Autodesk Inventor part; units mm, degrees
ref_plane "YZ Plane" through (0, 0, 0) normal (1, 0, 0) x (0, 1, 0)
ref_plane "XZ Plane" through (0, 0, 0) normal (0, 1, 0) x (-1, 0, 0)
ref_plane "XY Plane" through (0, 0, 0) normal (0, 0, 1) x (1, 0, 0)
sketch "Sketch1" plane through (0, 0, 0) normal (0, 1, 0) x (-1, 0, 0)
  line L0 (0, 0) -> (100, 0)
  line L1 (100, 0) -> (100, -110)
  line L2 (100, -110) -> (0, -110)
  line L3 (0, -110) -> (0, 0)
  line L4 (0, 0) -> (0, 0)
  line L5 (0, 0) -> (0, -150)
  line L6 (0, -150) -> (0, -150)
  line L7 (0, -150) -> (0, 0)
  line L8 (100, 0) -> (100, 0)
  line L9 (100, 0) -> (100, -150)
  line L10 (100, -150) -> (100, -150)
  line L11 (100, -150) -> (100, 0)
  point P0 (100, -110)
  point P1 (0, 0)
  point P2 (0, -110)
  dimension "d0" = 100
  dimension "d1" = 110
  dimension "d2" = 0
  dimension "d3" = 0
  dimension "d4" = 150
  dimension "d5" = 150
extrude "Extrusion1" add sketch "Sketch1" along normal blind 8
sketch "Sketch2" plane through (0, 8, 0) normal (0, 1, 0) x (1, 0, 0)
  circle A0 centre (-95, 5) radius 1.325
  line L0 (-100, 0) -> (0, 0)
  line L1 (-100, 110) -> (-100, 0)
  line L2 (-100, 55) -> (-85.0305, 55)
  line L3 (-50, 0) -> (-50, 9.4063)
  circle A1 centre (-95, 105) radius 1.325
  circle A2 centre (-5, 5) radius 1.325
  circle A3 centre (-5, 105) radius 1.325
  point P0 (0, 110)
  dimension "d118" = 5
  dimension "d119" = 5
  dimension "d120" = 2.65
extrude "Extrusion2" cut sketch "Sketch2" against normal blind 20
sketch "Sketch8" plane through (0, 8, 0) normal (0, 1, 0) x (1, 0, 0)
  line L0 (0, 0) -> (0, 110)
  arc A0 (-46.8357, 58.8714) -> (-46.1286, 58.1643) centre (-50, 55) ccw
  line L1 (-100, 0) -> (0, 0)
  line L2 (-55, 55) -> (-100, 55)
  line L3 (-100, 110) -> (-100, 0)
  line L4 (-50.2848, 59.9919) -> (-50.2848, 110)
  line L5 (0, 110) -> (-100, 110)
  circle A1 centre (-50, 55) radius 41
  circle A2 centre (-15, 55) radius 1.375
  circle A3 centre (-85, 55) radius 4
  line L6 (-50, 55) -> (-21.7157, 83.2843)
  line L7 (-46.8357, 58.8714) -> (-21.3643, 84.3428)
  line L8 (-46.1286, 58.1643) -> (-20.6572, 83.6357)
  line L9 (-47.688, 59.4333) -> (-22.7963, 84.325)
  line L10 (-45.5667, 57.312) -> (-20.675, 82.2037)
  arc A4 (-22.7963, 84.325) -> (-20.675, 82.2037) centre (-50, 55) ccw
  line L11 (-50, 55) -> (-21.7157, 26.7157)
  line L12 (-45.5667, 52.688) -> (-20.675, 27.7963)
  line L13 (-47.688, 50.5667) -> (-22.7963, 25.675)
  line L14 (-46.8357, 51.1286) -> (-21.3643, 25.6572)
  line L15 (-46.1286, 51.8357) -> (-20.6572, 26.3643)
  point P0 (-54.7697, 53.5)
  point P1 (-54.7697, 56.5)
  point P2 (-48.7848, 59.8501)
  point P3 (-21.3644, 27.0715)
  point P4 (-22.0715, 26.3644)
  dimension "d134" = 10
  dimension "d132" = 50
  dimension "d133" = 55
  dimension "d136" = 82
  dimension "d145" = 35
  dimension "d146" = 0
  dimension "d147" = 2.75
  dimension "d155" = 8
  dimension "d156" = 35
  dimension "d157" = 45
  dimension "d158" = 0.5
  dimension "d159" = 0.5
  dimension "d160" = 1
  dimension "d161" = 1
  dimension "d164" = 90
extrude "Extrusion5" cut sketch "Sketch8" against normal blind 20 contours A1 L7 A0 L9 A4 L4 | L4 A4 L2 A1 | L2 A4 L14 A1 | A1 L15 A4 L10 A0 L8 | A3 L2 | L2 A3 | L13 A0 L14 A4 | L15 A0 L12 A4 | A2
equation "\"d19\" = d18"
equation "\"d21\" = d22"
equation "\"BladeThickness\" = 1"
equation "\"NeckThickness\" = 1"
properties part number "FlexK7V2"
Check sheet for the modelled part. Datum: model origin and axes. Units: mm. A direction names the side the tool comes from. Round coordinates to 2 decimals unless told otherwise and drop trailing zeros. Order: outer loops, then holes, each group sorted by start corner. A loop starts at its lowest first (then second) coordinate and runs counter-clockwise, first axis right, second up.
Q1. Set-up check for faces 4 (the face through (0, 4, -56)), 5 (the face through (-34.278, 4.056, -71.429)): record each of +Z, -Z, +X, -X, +Y, -Y from which the full face is reachable in a straight line by a thin tool's end or side.
Filled sheet:
face 4: +Z, -Z, +X, +Y, -Y
face 5: +Y, -Y
Q2. Draft check along X on faces 1 (the face through (-49, 8, -54)), 2 (the face through (-33.3, 4.06, -69.58)), 3 (the face through (-100, 4, -54)). Enter one of: pulls with the +X half, pulls with the -X half, needs draft (parallel to the pull), parting line crosses it, or undercut.
Filled sheet:
face 1: needs draft
face 2: undercut
face 3: pulls with the -X half
Q3. Cross-section at B-B, the plane x = -5. Enter the section's corners in (y, z) (3 decimals), plus the area to 3 significant figures.
Filled sheet:
outline: (0, -110) - (8, -110) - (8, -106.325) - (0, -106.325) - close; (0, -103.675) - (8, -103.675) - (8, -6.325) - (0, -6.325) - close; (0, -3.675) - (8, -3.675) - (8, 0) - (0, 0) - close
area: 838 mm2
Q4. Cross-section at D-D, the plane y = 3. Give the number of separate pieces and of enclosed holes in the cut face, plus the area to 3 significant figures.
Filled sheet:
separate pieces: 1
enclosed holes: 8
area: 10,500 mm2
Q5. Cross-section at C-C, the plane z = -44. Enter the section's corners in (x, y), plus the area to 3 significant figures.
Filled sheet:
outline: (-100, 0) - (-89.5, 0) - (-89.5, 8) - (-100, 8) - close; (-88.46, 0) - (-41.12, 0) - (-41.12, 8) - (-88.46, 8) - close; (-39.71, 0) - (-38.29, 0) - (-38.29, 8) - (-39.71, 8) - close; (-36.88, 0) - (-11.54, 0) - (-11.54, 8) - (-36.88, 8) - close; (-10.5, 0) - (0, 0) - (0, 8) - (-10.5, 8) - close
area: 761 mm2
Q6. Cross-section at A-A, the plane z = -105. Enter the section's corners in (x, y) (3 decimals).
Filled sheet:
outline: (-100, 0) - (-96.325, 0) - (-96.325, 8) - (-100, 8) - close; (-93.675, 0) - (-6.325, 0) - (-6.325, 8) - (-93.675, 8) - close; (-3.675, 0) - (0, 0) - (0, 8) - (-3.675, 8) - close
Q7. Scan lines: L1, parallel to Z at x = -50, y = 5; L2, parallel to X at y = 5.75, z = -55 (3 decimals); L3, parallel to X at y = 3.25, z = -5 (3 decimals). Record each from-to range of solid material in increasing order.
Filled sheet:
L1: z = -110 to -96, -95 to -15, -14 to 0
L2: x = -100 to -91, -90 to -89, -81 to -16.375, -13.625 to -10, -9 to 0
L3: x = -100 to -96.325, -93.675 to -6.325, -3.675 to 0
